from build123d import *

# Parameters (mm, degrees)
SKETCH1_W           = 190.5
SKETCH1_H           = 95.25
BOSS_EXTRUDE1_DEPTH = 107.95
SKETCH2_R           = 8.255
CUT_EXTRUDE1_DEPTH  = 33.147


with BuildPart() as part:
    # Sketch1 → Boss-Extrude1 (new body)
    with BuildSketch(Plane(origin=(0, 0, 0), x_dir=(1, 0, 0), z_dir=(0, 1, 0))):
        with Locations((95.25, 47.625)):
            Rectangle(SKETCH1_W, SKETCH1_H)
    extrude(amount=BOSS_EXTRUDE1_DEPTH)

    # Sketch2 → Cut-Extrude1 (cut, symmetric)
    with BuildSketch(Plane(origin=(190.5, 0, 0), x_dir=(0, 0, -1), z_dir=(1, 0, 0))):
        with Locations((47.625, 53.286871915)):
            Circle(SKETCH2_R)
    extrude(amount=CUT_EXTRUDE1_DEPTH, both=True, mode=Mode.SUBTRACT)


solid = part.part
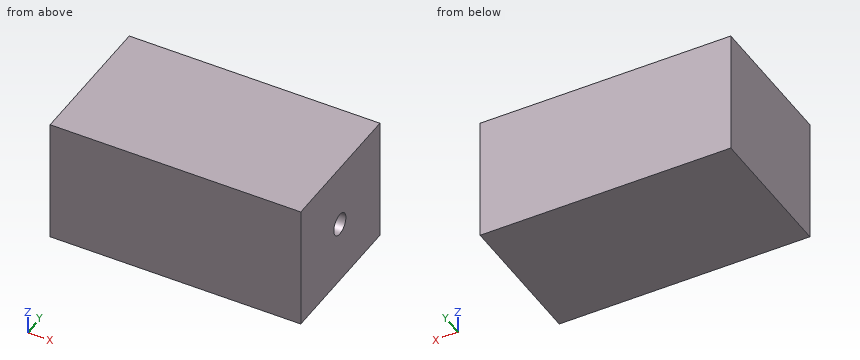
Check sheet for the modelled part. Datum: model origin and axes. Units: mm. Coordinates: 2 decimals unless noted, no trailing zeros. Loops run counter-clockwise (first coordinate to the right, second up) from the corner with the lowest first, then second, coordinate; pieces in that order, holes last. Notation, with made-up numbers: (80, 13) -> (105, 13) arc R31 cw to (105, 43) -> close; hole circle Ø8 at (44.5, -29). An arc over 180 degrees is marked (long way). Answer in a Markdown table with one row per item.
1. Sectioned sample at B-B, the plane z = -44. Record the boundary of the cut face in (x, y).
Check values:
| item | result |
|---|---|
| outline | (0, 0) -> (190.5, 0) -> (190.5, 45.87) -> (157.35, 45.87) -> (157.35, 60.7) -> (190.5, 60.7) -> (190.5, 107.95) -> (0, 107.95) -> close |
2. Sectioned sample at A-A, the plane y = 50.5. Record the boundary of the cut face in (x, z), then the cut area to 3 significant figures.
Check values:
| item | result |
|---|---|
| outline | (0, -95.25) -> (190.5, -95.25) -> (190.5, -55.4) -> (157.35, -55.4) -> (157.35, -39.85) -> (190.5, -39.85) -> (190.5, 0) -> (0, 0) -> close |
| area | 17,600 mm2 |
3. Go/stop test with flat-tipped pins: pin 1 (10 mm diameter, centred on x = 19.5, z = -68, fed in from -Y); pin 2 (13 mm diameter, centred on y = 53.29, z = -47.62, fed in from +X). Record where each tip stops, or that it passes through.
Check values:
| item | result |
|---|---|
| pin 1 | stops at y = 0 |
| pin 2 | stops at x = 157.35 |
